from build123d import *

# Parameters (mm, degrees)
SKETCH1_W           = 101.6
SKETCH1_H           = 127
BOSS_EXTRUDE1_DEPTH = 1.5875
SKETCH2_W           = 101.6
SKETCH2_H           = 127
SKETCH2_W_2         = 100.0125
SKETCH2_H_2         = 125.4125
EXTRUDE_THIN1_DEPTH = 50.8


with BuildPart() as part:
    # Sketch1 → Boss-Extrude1 (new body)
    with BuildSketch(Plane.XY):
        with Locations((-50.8, 63.5)):
            Rectangle(SKETCH1_W, SKETCH1_H)
    extrude(amount=BOSS_EXTRUDE1_DEPTH)

    # Sketch2 → Extrude-Thin1 (add)
    with BuildSketch(Plane.XY.offset(1.5875)):
        with Locations((-50.8, 63.5)):
            Rectangle(SKETCH2_W, SKETCH2_H)
        with Locations((-50.8, 63.5)):
            Rectangle(SKETCH2_W_2, SKETCH2_H_2, mode=Mode.SUBTRACT)
    extrude(amount=EXTRUDE_THIN1_DEPTH)


solid = part.part
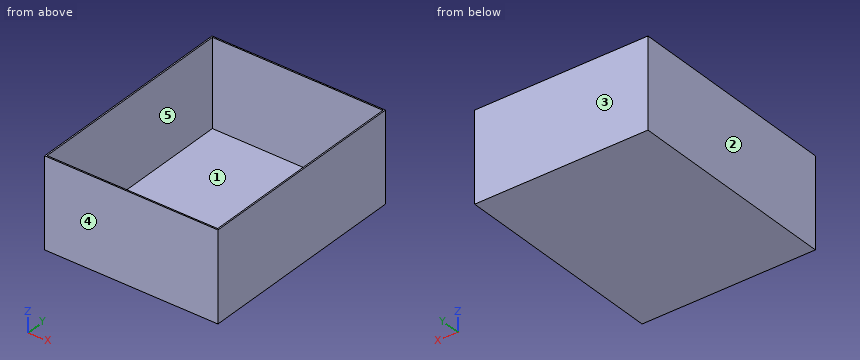
The listing builds one solid part. Answer for the finished solid, in the listing's coordinates (mm). Face numbers are marked on the shaded views. A direction names the side the tool comes from. Give positions to 0.01 mm unless a question says otherwise; leave off trailing zeros. Write each loop counter-clockwise with the first axis right and the second up, starting at its lowest first coordinate (ties: lowest second). Pieces come first, ordered by that corner, then holes.
Item 1: Which of the six approach directions +Z, -Z, +X, -X, +Y, -Y give full straight-line access (tool end or side, diameter ignored) to the marked faces 4 and 5?
Item 2: Determine the mould class of the marked faces 1, 2 and 3 for opening direction Y: released by +Y, released by -Y, zero draft, split by the parting line, or undercut.
Item 3: Find the intervals of material crossed by line 1 along X through (y, z) = (94, 17); line 2 along Y through (x, z) = (-14, 50.5); line 3 along Z through (x, y) = (-15, 71.5), in increasing order.
Item 4: A flat-ended cylindrical pin translates along its axis: P1, Ø6, axis at x = -77.5, y = 32, coming from the +Z side. Find the tip coordinate at first contact, or state that the pin passes through.
Item 5: Section B-B, the plane x = -73.5 is taken. Write down the section's boundary in (y, z), plus the area to 3 significant figures.
Item 6: Section A-A, the plane z = 40 is taken. Write down the section's boundary in (x, y), plus the area to 3 significant figures.
Item 7: Section C-C, the plane y = 85.5 is taken. Write down the section's boundary in (x, z), plus the area to 3 significant figures.
Completed:
1. face 4: +Z, -Z, +X, -X, -Y
1. face 5: +Z
2. face 1: undercut
2. face 2: zero draft
2. face 3: released by +Y
3. line 1: x = -101.6 to -100.81, -0.79 to 0
3. line 2: y = 0 to 0.79, 126.21 to 127
3. line 3: z = 0 to 1.59
4. P1: stops at z = 1.59
5. outline: (0, 0) - (127, 0) - (127, 52.39) - (126.21, 52.39) - (126.21, 1.59) - (0.79, 1.59) - (0.79, 52.39) - (0, 52.39) - close
5. area: 282 mm2
6. outline: (-101.6, 0) - (0, 0) - (0, 127) - (-101.6, 127) - close; hole (-100.81, 0.79) - (-0.79, 0.79) - (-0.79, 126.21) - (-100.81, 126.21) - close
6. area: 360 mm2
7. outline: (-101.6, 0) - (0, 0) - (0, 52.39) - (-0.79, 52.39) - (-0.79, 1.59) - (-100.81, 1.59) - (-100.81, 52.39) - (-101.6, 52.39) - close
7. area: 242 mm2
